Here's how the part is built. I have some questions about the finished solid (model axes, mm). A direction names the side the tool comes from. Give positions to 0.01 mm unless a question says otherwise; leave off trailing zeros. Loops run counter-clockwise (first coordinate to the right, second up) from the corner with the lowest first, then second, coordinate; pieces in that order, holes last. Notation, with made-up numbers: (28, 47) -> (84, 47) arc R21 cw to (84, 81) -> close; hole circle Ø7 at (81.5, 29). An arc over 180 degrees is marked (long way). Answer in a Markdown table with one row per item. Add a question column.
Item 1: If I drill on line 1 (Y direction, x = -11.1, z = 1.65); line 2 (Y direction, x = 11.1, z = 2.65); line 3 (X direction, y = 13, z = 3.4), over which ranges is the centre line in solid material (lowest first)?
Item 2: If we section it at C-C (z = 1): Write out the boundary of the cut face in (x, y), then the cut area to 3 significant figures.
Item 3: For P1, Ø1.5, axis at x = -8.5, y = -9, coming from the -Z side; P2, Ø0.6, axis at x = -2, z = 1, coming from the -Y side; P3, Ø1.5, axis at x = 0.5, z = 2, coming from the -Y side, each with a flat end and sliding along its axis, tell me the tip position at first contact or that it passes through.
Item 4: If we section it at B-B (y = -8.5): Write out the boundary of the cut face in (x, z), then the cut area to 3 significant figures.
Item 5: We'd pull the mould along Y, two halves only. Please class faces 4 (the face through (-13.4, 15.43, 2.03)), 5 (the face through (2.7, -5, 2)), 6 (the face through (0, 4, 4)): released by +Y, released by -Y, zero draft, split by the parting line, or undercut.
Item 6: Which directions (+Z, -Z, +X, -X, +Y, -Y) give clear straight access to the entire face, cutting with the end or side of a thin tool? Please do faces 1 (the face through (-2, -6.2, 2)), 2 (the face through (1.5, -9, 2)), 3 (the face through (0, 16, 2)).
Item 7: If we section it at A-A (x = 11.1): Write out the boundary of the cut face in (y, z), then the cut area to 3 significant figures.
Autodesk Inventor part; units mm, degrees
ref_plane "YZ Plane" through (0, 0, 0) normal (1, 0, 0) x (0, 1, 0)
ref_plane "XZ Plane" through (0, 0, 0) normal (0, 1, 0) x (-1, 0, 0)
ref_plane "XY Plane" through (0, 0, 0) normal (0, 0, 1) x (1, 0, 0)
sketch "Sketch1" plane through (0, 0, 0) normal (0, 0, 1) x (1, 0, 0)
  line L0 (-14, 0) -> (14, 0)
  line L1 (14, 0) -> (14, 16)
  line L2 (14, 16) -> (-14, 16)
  line L3 (-14, 16) -> (-14, 0)
  circle A0 centre (-11.1, 2.85) radius 1.55
  circle A1 centre (11.1, 13.15) radius 1.55
  line L4 (-11.1, 2.85) -> (-14, 2.85) construction
  line L5 (11.1, 13.15) -> (14, 13.15) construction
  line L6 (11.1, 13.15) -> (11.1, 16) construction
  line L7 (-11.1, 2.85) -> (-11.1, 0) construction
  line L8 (-14, 0) -> (14, 0) construction
  line L9 (14, 0) -> (14, -11)
  line L10 (14, -11) -> (8, -11) construction
  line L11 (-14, -11) -> (-14, 0)
  line L12 (-14, -11) -> (-8, -11) construction
  line L13 (-8, -11) -> (-8, -15)
  line L14 (-8, -15) -> (-14, -15)
  line L15 (-14, -15) -> (-14, -11)
  line L16 (14, -11) -> (8, -11) construction
  line L17 (8, -11) -> (8, -15)
  line L18 (8, -15) -> (14, -15)
  line L19 (14, -15) -> (14, -11)
  line L20 (-8, -11) -> (-14, -11) construction
  line L21 (8, -11) -> (-8, -11)
  point P0 (0, 0)
  point P1 (0, 0)
  point P2 (14, 0)
  point P3 (14, 0)
  dimension "d0" = 3.1
  dimension "d1" = 22.2
  dimension "d2" = 10.3
  dimension "d3" = 16
  dimension "d4" = 28
  dimension "d5" = 27
  dimension "d8" = 6
  dimension "d9" = 6
  dimension "d10" = 4
extrude "Extrusion1" add sketch "Sketch1" along normal blind 4
sketch "Sketch2" plane through (0, 0, 0) normal (0, 0, -1) x (-1, 0, 0)
  line L0 (8, -11) -> (-8, -11)
  line L1 (-1.5, -11) -> (1.5, -11)
  line L2 (1.5, -11) -> (1.5, 1)
  line L3 (1.5, 1) -> (-1.5, 1)
  line L4 (-1.5, 1) -> (-1.5, -11)
  line L5 (-2.7, -6.2) -> (2.7, -6.2)
  line L6 (2.7, -6.2) -> (2.7, -3.8)
  line L7 (2.7, -3.8) -> (-2.7, -3.8)
  line L8 (-2.7, -3.8) -> (-2.7, -6.2)
  point P0 (0, 0)
  point P1 (-2.7, -5)
  point P2 (-1.5, -5)
  point P3 (0, -3.8)
  point P4 (0, 1)
  point P5 (0, -11)
  point P6 (0, -11)
  point P7 (-1.5, -6.2)
  point P8 (1.5, -6.2)
  point P9 (1.5, -3.8)
  point P10 (-1.5, -3.8)
  dimension "d11" = 3
  dimension "d12" = 12
  dimension "d13" = 5.4
  dimension "d14" = 2.4
extrude "Extrusion2" cut sketch "Sketch2" against normal up to next
fillet "Fillet1" radius 2 2 edges at (14, 16, 2) (-14, 16, 2)
properties part number "SwitchHolder_V2" material "MDF Medium Density Fiberboard"
Recorded:
| question | item | result |
|---|---|---|
| 1 | line 1 | y = -15 to 1.3, 4.4 to 16 |
| 1 | line 2 | y = -15 to 11.6, 14.7 to 16 |
| 1 | line 3 | x = -14 to 9.56, 12.64 to 14 |
| 2 | outline | (-14, -15) -> (-8, -15) -> (-8, -11) -> (-1.5, -11) -> (-1.5, -6.2) -> (-2.7, -6.2) -> (-2.7, -3.8) -> (-1.5, -3.8) -> (-1.5, 1) -> (1.5, 1) -> (1.5, -3.8) -> (2.7, -3.8) -> (2.7, -6.2) -> (1.5, -6.2) -> (1.5, -11) -> (8, -11) -> (8, -15) -> (14, -15) -> (14, 14) arc R2 ccw to (12, 16) -> (-12, 16) arc R2 ccw to (-14, 14) -> close; hole circle Ø3.1 at (-11.1, 2.85); hole circle Ø3.1 at (11.1, 13.15) |
| 2 | area | 745 mm^2 |
| 3 | P1 | stops at z = 0 |
| 3 | P2 | stops at y = -11 |
| 3 | P3 | stops at y = 1 |
| 4 | outline | (-14, 0) -> (-1.5, 0) -> (-1.5, 4) -> (-14, 4) -> close; (1.5, 0) -> (14, 0) -> (14, 4) -> (1.5, 4) -> close |
| 4 | area | 100 mm^2 |
| 5 | face 4 | released by +Y |
| 5 | face 5 | undercut |
| 5 | face 6 | zero draft |
| 6 | face 1 | +Z, -Z |
| 6 | face 2 | +Z, -Z, -Y |
| 6 | face 3 | +Z, -Z, +X, -X, +Y |
| 7 | outline | (-15, 0) -> (11.6, 0) -> (11.6, 4) -> (-15, 4) -> close; (14.7, 0) -> (16, 0) -> (16, 4) -> (14.7, 4) -> close |
| 7 | area | 112 mm^2 |
